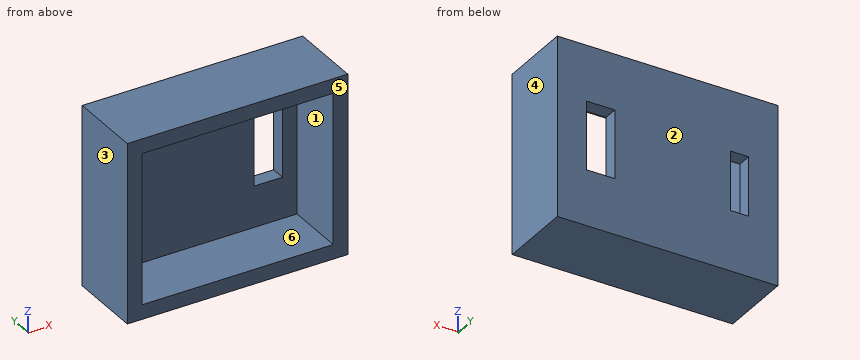
Autodesk Inventor part; units mm, degrees
ref_plane "YZ Plane" through (0, 0, 0) normal (1, 0, 0) x (0, 1, 0)
ref_plane "XZ Plane" through (0, 0, 0) normal (0, 1, 0) x (-1, 0, 0)
ref_plane "XY Plane" through (0, 0, 0) normal (0, 0, 1) x (1, 0, 0)
sketch "Sketch1" plane through (0, 0, 0) normal (0, 1, 0) x (-1, 0, 0)
  line L0 (0, 0) -> (41.91, 0)
  line L1 (41.91, 0) -> (41.91, -33.02)
  line L2 (41.91, -33.02) -> (0, -33.02)
  line L3 (0, -33.02) -> (0, 0)
  line L4 (41.91, -16.51) -> (34.735, -16.51)
  line L5 (34.735, -16.51) -> (34.735, -10.01)
  line L6 (34.735, -10.01) -> (41.91, -10.01)
  line L7 (34.735, -10.01) -> (38.735, -10.01)
  line L8 (38.735, -10.01) -> (38.735, -23.01)
  line L9 (38.735, -23.01) -> (34.735, -23.01)
  line L10 (34.735, -23.01) -> (34.735, -10.01)
  line L11 (0, -16.51) -> (9.425, -16.51)
  line L12 (9.425, -16.51) -> (9.425, -9.01)
  line L13 (9.425, -9.01) -> (3.175, -9.01)
  line L14 (3.175, -9.01) -> (3.175, -24.01)
  line L15 (3.175, -24.01) -> (9.425, -24.01)
  line L16 (9.425, -24.01) -> (9.425, -9.01)
  point P0 (0, -9.01)
  point P1 (0, -24.01)
  point P2 (41.91, -23.01)
  point P3 (3.175, -16.51)
  point P4 (38.735, -16.51)
  dimension "d0" = 41.91
  dimension "d1" = 33.02
  dimension "d2" = 7.175
  dimension "d3" = 6.5
  dimension "d4" = 4
  dimension "d5" = 13
  dimension "d6" = 9.425
  dimension "d7" = 7.5
  dimension "d8" = 6.25
  dimension "d9" = 15
extrude "Extrusion1" add sketch "Sketch1" along normal blind 3.175 contours L0 L1 L6 L5 L10 L9 L8 L4 L2 L3 | L1 L4 L8 L6
sketch "Sketch2" plane through (0, 3.175, 0) normal (0, 1, 0) x (1, 0, 0)
  line L0 (0, 0) -> (0, 33.02)
  line L1 (-3.175, 9.01) -> (-9.425, 9.01)
  line L2 (-9.425, 9.01) -> (-9.425, 24.01)
  line L3 (-9.425, 24.01) -> (-3.175, 24.01)
  line L4 (0, 33.02) -> (-41.91, 33.02)
  line L5 (-41.91, 33.02) -> (-41.91, 0)
  line L6 (-38.735, 23.01) -> (-34.735, 23.01)
  line L7 (-34.735, 23.01) -> (-34.735, 10.01)
  line L8 (-41.91, 0) -> (0, 0)
  line L9 (3.175, -3.175) -> (3.175, 12.185)
  line L10 (3.175, 12.185) -> (-6.25, 12.185)
  line L11 (-6.25, 12.185) -> (-6.25, 20.835)
  line L12 (-6.25, 20.835) -> (3.175, 20.835)
  line L13 (3.175, 20.835) -> (3.175, 36.195)
  line L14 (3.175, 36.195) -> (-45.085, 36.195)
  line L15 (-45.085, 36.195) -> (-45.085, 19.835)
  line L16 (-45.085, 19.835) -> (-37.91, 19.835)
  line L17 (-37.91, 19.835) -> (-37.91, 13.185)
  line L18 (-37.91, 13.185) -> (-45.085, 13.185)
  line L19 (-45.085, 13.185) -> (-45.085, -3.175)
  line L20 (-45.085, -3.175) -> (3.175, -3.175)
  line L21 (3.175, 12.185) -> (3.175, 20.835)
  line L22 (0, 24.01) -> (0, 9.01)
  line L23 (-41.91, 10.01) -> (-41.91, 23.01)
  line L24 (-45.085, 19.835) -> (-45.085, 13.185)
  line L25 (-3.175, 24.01) -> (-3.175, 9.01)
  line L26 (-38.735, 10.01) -> (-38.735, 23.01)
  line L27 (-34.735, 10.01) -> (-38.735, 10.01)
  point P0 (-41.91, 19.835)
  point P1 (0, 20.835)
  point P2 (-3.175, 20.835)
  point P3 (-3.175, 12.185)
  point P4 (0, 12.185)
  point P5 (-41.91, 13.185)
  point P6 (-38.735, 13.185)
  point P7 (-38.735, 19.835)
  dimension "d12" = 3.175
extrude "Extrusion2" add sketch "Sketch2" against normal blind 16.1648 contours L0 L10 L9 L20 L19 L18 L5 L8 | L0 L12 L21 L10 | L0 L4 L5 L16 L15 L14 L13 L12 | L18 L24 L16 L5
properties part number "pololuCaseTop"
The listing builds one solid part. Answer for the finished solid, in the listing's coordinates (mm). Face numbers are marked on the shaded views. A direction names the side the tool comes from. Give positions to 0.01 mm unless a question says otherwise; leave off trailing zeros. Order: outer loops, then holes, each group sorted by start corner. A loop starts at its lowest first (then second) coordinate and runs counter-clockwise, first axis right, second up. Notation, with made-up numbers: (-7.5, 28) -> (38.5, 28) arc R21 ccw to (38.5, 58) -> close; hole circle Ø2 at (-6.75, 41.25). An arc over 180 degrees is marked (long way). Answer as a JSON object with one key per item and string values. Group by question number.
Item 1: The part is cut by section B-B on z = -16. Write down the section's boundary in (x, y) (3 decimals), and give its area (3 significant figures).
Item 2: A flat-ended cylindrical pin translates along its axis: pin 1 (12 mm diameter, centred on x = -17, z = -29, fed in from -Y). Find the tip coordinate at first contact, or state that the pin passes through.
Item 3: Determine the mould class of the marked faces 1, 2, 3 and 4 for opening direction X: pulls with the +X half, pulls with the -X half, needs draft (parallel to the pull), parting line crosses it, or undercut.
Item 4: A tool of negligible diameter and unlimited length cuts with its end or side. For the marked faces 5 and 6, from which of +Z, -Z, +X, -X, +Y, -Y can it reach the whole face along a straight path? Write none if from no direction.
Item 5: The part is cut by section D-D on z = -5. Write down the section's boundary in (x, y) (3 decimals), and give its area (3 significant figures).
Item 6: The part is cut by section A-A on y = -11. Write down the section's boundary in (x, z) (3 decimals).
Item 7: Consider L1, parallel to Z at x = -38.5, y = -5 (3 decimals); L2, parallel to X at y = -2.5, z = -15 (3 decimals); L3, parallel to Y at x = -15, z = -25.5 (3 decimals). Determine where each line is inside the solid, lowest interval first. Write a range as from..to.
Item 8: The part is cut by section C-C on x = -1. Write down the section's boundary in (y, z) (3 decimals), and give its area (3 significant figures).
Result set:
{
 "1": {"outline": "(-45.085, -12.99) -> (-41.91, -12.99) -> (-41.91, 0) -> (-38.735, 0) -> (-38.735, 3.175) -> (-45.085, 3.175) -> close; (-34.735, 0) -> (-9.425, 0) -> (-9.425, 3.175) -> (-34.735, 3.175) -> close; (-3.175, 0) -> (0, 0) -> (0, -12.99) -> (3.175, -12.99) -> (3.175, 3.175) -> (-3.175, 3.175) -> close", "area": "203 mm²"},
 "2": {"pin 1": "y = -12.99"},
 "3": {"face 1": "undercut", "face 2": "needs draft", "face 3": "pulls with the -X half", "face 4": "pulls with the +X half"},
 "4": {"face 5": "+Z, -Z, +X, -X, -Y", "face 6": "-Y"},
 "5": {"outline": "(-45.085, -12.99) -> (-41.91, -12.99) -> (-41.91, 0) -> (0, 0) -> (0, -12.99) -> (3.175, -12.99) -> (3.175, 3.175) -> (-45.085, 3.175) -> close", "area": "236 mm²"},
 "6": {"outline": "(-45.085, -36.195) -> (3.175, -36.195) -> (3.175, 3.175) -> (-45.085, 3.175) -> close; hole (-41.91, -33.02) -> (0, -33.02) -> (0, 0) -> (-41.91, 0) -> close"},
 "7": {"L1": "-36.195..-33.02, 0..3.175", "L2": "-45.085..-41.91, 0..3.175", "L3": "0..3.175"},
 "8": {"outline": "(-12.99, -36.195) -> (3.175, -36.195) -> (3.175, 3.175) -> (-12.99, 3.175) -> (-12.99, 0) -> (0, 0) -> (0, -33.02) -> (-12.99, -33.02) -> close", "area": "207 mm²"}
}
